```python
from build123d import *

# Parameters (mm, degrees)
EXTRUDE_1_DEPTH      = 5
EXTRUDE_1_DEPTH_BACK = 5
SKETCH_367_W         = 9
SKETCH_367_H         = 2
FILLET_1_R           = 5
FILLET_2_R           = 1
SKETCH_1_R           = 1.75
CUT_EXTRUDE_2_DEPTH  = 29.731515797
SKETCH_1_6_R         = 3
CUT_EXTRUDE_3_DEPTH  = 1
SKETCH_5_W           = 10
SKETCH_5_H           = 10
EXTRUDE_2_DEPTH      = 2
SKETCH_6_R           = 1.75
CUT_EXTRUDE_5_DEPTH  = 24.963513933
SKETCH_6_3_R         = 3
CUT_EXTRUDE_6_DEPTH  = 11
CUT_EXTRUDE_7_DEPTH  = 1


with BuildPart() as part:
    # Sketch 367 → Бобышка-Вытянуть1 (new, two sides: drawn at the far end of the back side and taken through both)
    with BuildSketch(Plane.XY.offset(-EXTRUDE_1_DEPTH_BACK)):
        with BuildLine():
            ThreePointArc((-7.348469228, 10.723805295), (13, 0), (-7.348469228, -10.723805295))
            Line((-7.348469228, -10.723805295), (-10.5, -7.5))
            Line((-10.5, -7.5), (-10.5, -5.5))
            Line((-10.5, -5.5), (-7.348469228, -7.5))
            ThreePointArc((-7.348469228, -7.5), (10.5, 0), (-7.348469228, 7.5))
            Line((-7.348469228, 7.5), (-10.5, 5.5))
            Line((-10.5, 5.5), (-10.5, 7.5))
            Line((-10.5, 7.5), (-7.348469228, 10.723805295))
        make_face()
        with Locations((-15, 6.5)):
            Rectangle(SKETCH_367_W, SKETCH_367_H)
        with Locations((-15, -6.5)):
            Rectangle(SKETCH_367_W, SKETCH_367_H)
    extrude(amount=EXTRUDE_1_DEPTH + EXTRUDE_1_DEPTH_BACK)

    # Скругление1
    fillet_1_edges = [part.edges().sort_by_distance(p)[0] for p in [
        (-7.348469228, -10.723805295, 0),
        (-10.5, -7.5, 0),
        (-10.5, -5.5, 0),
        (-7.348469228, -7.5, 0),
        (-7.348469228, 7.5, 0),
        (-10.5, 5.5, 0),
        (-10.5, 7.5, 0),
        (-7.348469228, 10.723805295, 0),
    ]]
    fillet(fillet_1_edges, radius=FILLET_1_R)

    # Скругление2
    fillet_2_edges = [part.edges().sort_by_distance(p)[0] for p in [
        (-19.5, -7.5, 0),
        (-19.5, -5.5, 0),
        (-19.5, 5.5, 0),
        (-19.5, 7.5, 0),
    ]]
    fillet(fillet_2_edges, radius=FILLET_2_R - 0.0001)  # a hair under: the kernel refuses the full size

    # Эскиз1 → Вырез-Вытянуть2 (cut, through all)
    with BuildSketch(Plane(origin=(0, 7.5, 0), x_dir=(1, 0, 0), z_dir=(0, 1, 0))):
        with Locations(Location((-15.5, 0, 0), (0, 0, 270))):
            Circle(SKETCH_1_R)
    extrude(amount=-CUT_EXTRUDE_2_DEPTH, mode=Mode.SUBTRACT)

    # Эскиз1<6> → Вырез-Вытянуть3 (cut)
    with BuildSketch(Plane(origin=(0, 7.5, 0), x_dir=(1, 0, 0), z_dir=(0, 1, 0))):
        with Locations(Location((-15.5, 0, 0), (0, 0, 270))):
            Circle(SKETCH_1_6_R)
    extrude(amount=-CUT_EXTRUDE_3_DEPTH, mode=Mode.SUBTRACT)

    # Эскиз5 → Бобышка-Вытянуть2 (add)
    with BuildSketch(Plane(origin=(13, 0, 0), x_dir=(0, 0, -1), z_dir=(1, 0, 0))):
        Rectangle(SKETCH_5_W, SKETCH_5_H)
    extrude(amount=-EXTRUDE_2_DEPTH)

    # Эскиз6 → Вырез-Вытянуть5 (cut, through all)
    with BuildSketch(Plane(origin=(0, 0, 0), x_dir=(0, 0, -1), z_dir=(1, 0, 0))):
        with Locations(Location((0, 0, 0), (0, 0, 180))):
            Circle(SKETCH_6_R)
    extrude(amount=CUT_EXTRUDE_5_DEPTH, mode=Mode.SUBTRACT)

    # Эскиз6<3> → Вырез-Вытянуть6 (cut)
    with BuildSketch(Plane(origin=(0, 0, 0), x_dir=(0, 0, -1), z_dir=(1, 0, 0))):
        with Locations(Location((0, 0, 0), (0, 0, 180))):
            Circle(SKETCH_6_3_R)
    extrude(amount=CUT_EXTRUDE_6_DEPTH, mode=Mode.SUBTRACT)

    # Эскиз8 → Вырез-Вытянуть7 (cut)
    with BuildSketch(Plane.XZ.offset(7.5)):
        Polygon((-15.5, 3.464101615), (-18.5, 1.732050808), (-18.5, -1.732050808), (-15.5, -3.464101615), (-12.5, -1.732050808), (-12.5, 1.732050808), align=None)
    extrude(amount=-CUT_EXTRUDE_7_DEPTH, mode=Mode.SUBTRACT)


solid = part.part
```
Check sheet for the modelled part. Datum: model origin and axes. Units: mm. A direction names the side the tool comes from. Round coordinates to 2 decimals unless told otherwise and drop trailing zeros. Loops run counter-clockwise (first coordinate to the right, second up) from the corner with the lowest first, then second, coordinate; pieces in that order, holes last. Notation, with made-up numbers: M 71.25,36 L 79.25,36 A15 cw 79.25,47 Z; hole C -8.75,69.5 d8. An arc over 180 degrees is marked long. Answer as a JSON object with one key per item and string values.
1. Gauge pin test, flat ends, axial feed: P1, Ø1.1, axis at x = 12.5, z = 0, coming from the +Y side; P2, Ø2, axis at x = -4, y = 7.5, coming from the -Z side; P3, Ø3, axis at x = -16, z = -2.5, coming from the +Y side; P4, Ø0.5, axis at y = -7, z = 0, coming from the -X side. Record the tip position at first contact, or that the pin passes through.
Reply:
{"P1": "stops at y = 5.12", "P2": "passes through", "P3": "stops at y = 7.5", "P4": "stops at x = -19.47"}
2. Section check D-D (z = 0). State how many separate pieces and enclosed holes the cut face has, plus the area to 3 significant figures.
Reply:
{"separate pieces": "4", "enclosed holes": "0", "area": "158 mm²"}
3. Mould release check, pull along Y, two halves, no side actions. Record for faces 1 (the flat face through (-13.8, -5.5, -1.2)), 2 (the cylindrical face through (-7.263, -10.753, 0.07)), 3 (the flat face through (-18.5, -7, 0)): pulls with the +Y half, pulls with the -Y half, needs draft (parallel to the pull), parting line crosses it, or undercut.
Reply:
{"face 1": "undercut", "face 2": "pulls with the -Y half", "face 3": "needs draft"}
4. Section check C-C (x = -16). Record the boundary of the cut face in (y, z).
Reply:
{"outline": "M -7.5,-5 L -5.5,-5 L -5.5,-1.68 L -6.5,-1.68 L -6.5,-3.18 L -7.5,-3.18 Z; M -7.5,3.18 L -6.5,3.18 L -6.5,1.68 L -5.5,1.68 L -5.5,5 L -7.5,5 Z; M 5.5,-5 L 7.5,-5 L 7.5,-2.96 L 6.5,-2.96 L 6.5,-1.68 L 5.5,-1.68 Z; M 5.5,1.68 L 6.5,1.68 L 6.5,2.96 L 7.5,2.96 L 7.5,5 L 5.5,5 Z"}
5. Scan lines: line 1 (Z direction, x = -15.5, y = 7); line 2 (Y direction, x = -14, z = -1); line 3 (X direction, y = -8.25, z = -0.5). Record each from-to range of solid material in increasing order.
Reply:
{"line 1": "z = -5 to -3, 3 to 5", "line 2": "y = -6.5 to -5.5, 5.5 to 6.5", "line 3": "x = -9.97 to -6.5, 6.5 to 10.05"}
6. Section check B-B (x = 0). Record the boundary of the cut face in (y, z), plus the area to 3 significant figures.
Reply:
{"outline": "M -13,-5 L -10.5,-5 L -10.5,5 L -13,5 Z; M 10.5,-5 L 13,-5 L 13,5 L 10.5,5 Z", "area": "50.0 mm²"}
7. Section check A-A (y = 0). Record the boundary of the cut face in (x, z), plus the area to 3 significant figures.
Reply:
{"outline": "M 10.5,-5 L 13,-5 L 13,-1.75 L 11,-1.75 L 11,-3 L 10.5,-3 Z; M 10.5,3 L 11,3 L 11,1.75 L 13,1.75 L 13,5 L 10.5,5 Z", "area": "15.0 mm²"}
8. Access from +Z, -Z, +X, -X, +Y, -Y to the whole of each face (thin tool, end or side, straight path). Record for faces 4 (the cylindrical face through (10.62, -2.03, -2.21)), 5 (the flat face through (-8.522, -6.755, -0.07)), 6 (the flat face through (-17, -7, -2.6)).
Reply:
{"face 4": "-X", "face 5": "+Z, -Z", "face 6": "-Y"}
